Build history of the part. All positions in model axes, mm. Face numbers are marked on the shaded views. A direction names the side the tool comes from. Round coordinates to 2 decimals unless told otherwise and drop trailing zeros. Write each loop counter-clockwise with the first axis right and the second up, starting at its lowest first coordinate (ties: lowest second). Pieces come first, ordered by that corner, then holes. Notation, with made-up numbers: (29, 39.5) -> (61, 39.5) arc R24 cw to (61, 50.5) -> close; hole circle Ø5 at (-21, 20). An arc over 180 degrees is marked (long way). Return JSON: item names as keys, results as strings.
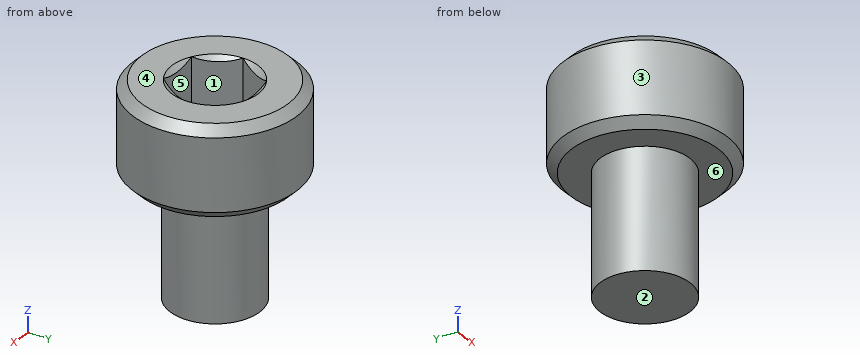
from build123d import *

# Parameters (mm, degrees)
F3_DEPTH = 2
F6_SIZE  = 0.3


with BuildPart() as f1:
    # F0 (on Front) → F1 (revolve)
    with BuildSketch(Plane.XZ):
        Polygon((2.75, 3), (0, 3), (0, -4), (1.5, -4), (1.5, 0), (2.75, 0), align=None)
    revolve(axis=Axis((0, 0, -0.5), (0, 0, -1)))

    # F2 (on face) → F3 (cut)
    with BuildSketch(Plane.XY.offset(3)):
        Polygon((1.443375673, 0), (0.7216878365, 1.25), (-0.7216878365, 1.25), (-1.443375673, 0), (-0.7216878365, -1.25), (0.7216878365, -1.25), align=None)
    extrude(amount=-F3_DEPTH, mode=Mode.SUBTRACT)

    # F4 (on Front) → F5 (revolve, cut)
    with BuildSketch(Plane.XZ):
        with BuildLine():
            Line((0, 2.5), (0, 7.1666666667))
            ThreePointArc((0, 7.1666666667), (-2.3333333333, 4.8333333333), (0, 2.5))
        make_face()
    revolve(axis=Axis((0, 0, 2.4166666667), (0, 0, -1)), mode=Mode.SUBTRACT)

    # F6
    f6_edges = [f1.edges().sort_by_distance(p)[0] for p in [
        (-2.75, 0, 3),
        (-2.75, 0, 0),
    ]]
    chamfer(f6_edges, length=F6_SIZE)


solid = f1.part
Q1. Wall check: L1, parallel to Z at x = -0.7, y = 0.45; L2, parallel to Z at x = -2.1, y = -0.3; L3, parallel to X at y = -1.2, z = 1.5. Give the ranges that are in metal, low to high.
Verdict:
{"L1": "z = -4 to 1", "L2": "z = 0 to 3", "L3": "x = -2.47 to -0.75, 0.75 to 2.47"}
Q2. Two-plate mould, pull along Y, no slides. Class the marked faces 1, 2 and 3: +Y half, -Y half, draft (parallel to the pull), parting line (faces both ways), or undercut.
Verdict:
{"face 1": "undercut", "face 2": "draft", "face 3": "parting line"}
Q3. Saw through at B-B on x = 0. List the corners of the cut face in (y, z).
Verdict:
{"outline": "(-2.75, 0.3) -> (-2.45, 0) -> (-1.5, 0) -> (-1.5, -4) -> (1.5, -4) -> (1.5, 0) -> (2.45, 0) -> (2.75, 0.3) -> (2.75, 2.7) -> (2.45, 3) -> (1.44, 3) arc R2.33 cw to (1.25, 2.86) -> (1.25, 1) -> (-1.25, 1) -> (-1.25, 2.86) arc R2.33 cw to (-1.44, 3) -> (-2.45, 3) -> (-2.75, 2.7) -> close"}
Q4. Saw through at C-C on z = 0.5. List the corners of the cut face in (x, y).
Verdict:
{"outline": "circle Ø5.5 at (0, 0)"}
Q5. 3-axis set-ups, long thin cutter, end or side, ignore diameter. For the marked faces 4, 5 and 6: which of +Z, -Z, +X, -X, +Y, -Y reach the whole face in a straight line?
Verdict:
{"face 4": "+Z, +X, -X, +Y, -Y", "face 5": "+Z", "face 6": "-Z"}
Q6. Saw through at A-A on z = 2.25. List the corners of the cut face in (x, y), then the cut area to 3 significant figures.
Verdict:
{"outline": "circle Ø5.5 at (0, 0); hole (-1.44, 0) -> (-0.72, -1.25) -> (0.72, -1.25) -> (1.44, 0) -> (0.72, 1.25) -> (-0.72, 1.25) -> close", "area": "18.3 mm²"}
Q7. Saw through at D-D on z = -2. List the corners of the cut face in (x, y).
Verdict:
{"outline": "circle Ø3 at (0, 0)"}
Q8. Pin check, flat tips, straight feed: pin 1 Ø0.8 at (x, y) = (-0.5, 0) entering from +Z; pin 2 Ø3 at (x, z) = (1.5, -3) entering from +Y. Stop position of each tip, or through.
Verdict:
{"pin 1": "stops at z = 1", "pin 2": "stops at y = 1.5"}
